```python
from build123d import *

# Parameters (mm, degrees)
F0_R     = 12.5
F0_R_2   = 2.55
F1_DEPTH = 6


# Not quite as in the source:
# - ends of sketch curves that miss each other by under 0.0002 mm in the source are joined


with BuildPart() as f1:
    # F0 (on Top) → F1 (new body)
    with BuildSketch(Plane.XY):
        with BuildLine():
            Line((38, 19.75), (-38, 19.75))
            ThreePointArc((-38, 19.75), (-40.1213203436, 18.8713203436), (-41, 16.75))
            Line((-41, 16.75), (-41, -16.75))
            ThreePointArc((-41, -16.75), (-40.1213203436, -18.8713203436), (-38, -19.75))
            Line((-38, -19.75), (38, -19.75))
            ThreePointArc((38, -19.75), (40.1213203436, -18.8713203436), (41, -16.75))
            Line((41, -16.75), (41, 16.75))
            ThreePointArc((41, 16.75), (40.1213203436, 18.8713203436), (38, 19.75))
        make_face()
        with BuildLine():
            ThreePointArc((-34.1539839892, -16.5960150108), (-36.3460155108, -16.5960155108), (-36.3460150108, -14.4039839892))
            Line((-36.346015, -14.403984), (-33.846015, -11.903984))
            ThreePointArc((-33.8460150108, -11.9039839892), (-31.6539844892, -11.9039844892), (-31.6539839892, -14.0960150108))
            Line((-31.653984, -14.096015), (-34.153984, -16.596015))
        make_face(mode=Mode.SUBTRACT)
        with BuildLine():
            ThreePointArc((-3.1539844892, -14.4039844892), (-3.1539844892, -16.5960155108), (-5.3460155108, -16.5960155108))
            Line((-5.3460155108, -16.5960155108), (-7.846015, -14.096015))
            ThreePointArc((-7.846015, -14.096015), (-7.8460155108, -11.9039844892), (-5.6539844892, -11.9039844892))
            Line((-5.6539844892, -11.9039844892), (-3.1539844892, -14.4039844892))
        make_face(mode=Mode.SUBTRACT)
        with Locations((-19.25, 0)):
            Circle(F0_R, mode=Mode.SUBTRACT)
        with Locations((12.8, -10)):
            Circle(F0_R_2, mode=Mode.SUBTRACT)
        with Locations((32.8, -10)):
            Circle(F0_R_2, mode=Mode.SUBTRACT)
        with Locations((12.8, 0)):
            Circle(F0_R_2, mode=Mode.SUBTRACT)
        with Locations((32.8, 0)):
            Circle(F0_R_2, mode=Mode.SUBTRACT)
        with BuildLine():
            ThreePointArc((-31.6539844892, 14.0960155108), (-31.6539844892, 11.9039844892), (-33.8460155108, 11.9039844892))
            Line((-33.8460155108, 11.9039844892), (-36.346015, 14.403985))
            ThreePointArc((-36.346015, 14.403985), (-36.3460155108, 16.5960155108), (-34.1539844892, 16.5960155108))
            Line((-34.1539844892, 16.5960155108), (-31.6539844892, 14.0960155108))
        make_face(mode=Mode.SUBTRACT)
        with BuildLine():
            ThreePointArc((-5.3460150108, 16.5960160108), (-3.1539844892, 16.5960155108), (-3.1539839892, 14.4039849892))
            Line((-3.153984, 14.403985), (-5.653984, 11.903985))
            ThreePointArc((-5.6539839892, 11.9039849892), (-7.8460155108, 11.9039844892), (-7.8460150108, 14.0960160108))
            Line((-7.846015, 14.096016), (-5.346015, 16.596016))
        make_face(mode=Mode.SUBTRACT)
        with Locations((12.8, 10)):
            Circle(F0_R_2, mode=Mode.SUBTRACT)
        with Locations((32.8, 10)):
            Circle(F0_R_2, mode=Mode.SUBTRACT)
    extrude(amount=F1_DEPTH)


solid = f1.part
```
Could you check a few things on this model? Use its own coordinates, in mm. A direction names the side the tool comes from. Round coordinates to 2 decimals unless told otherwise and drop trailing zeros. Loops run counter-clockwise (first coordinate to the right, second up) from the corner with the lowest first, then second, coordinate; pieces in that order, holes last. Notation, with made-up numbers: (-33.75, 45) -> (9.25, 45) arc R20 cw to (9.25, 79) -> close; hole circle Ø4 at (-37.5, 26.25). An arc over 180 degrees is marked (long way). One line per question, with ' | ' between items.
(1) For faces 1 (the face through (-4.42, -13.14, 2.96)), 2 (the face through (1, 19.75, 3)), which set-ups out of +Z, -Z, +X, -X, +Y, -Y let a thin tool reach every point of the face, with its end or its side?
Model answer:
face 1: +Z, -Z | face 2: +Z, -Z, +X, -X, +Y
(2) If we section it at D-D on x = -19.25: List the corners of the cut face in (y, z) for me, and give its area (3 significant figures).
Model answer:
outline: (-19.75, 0) -> (-12.5, 0) -> (-12.5, 6) -> (-19.75, 6) -> close; (12.5, 0) -> (19.75, 0) -> (19.75, 6) -> (12.5, 6) -> close | area: 87.0 mm^2
(3) Thinking about a two-plate mould opening in X: for faces 3 (the face through (-6.58, -15.36, 2.96)), 4 (the face through (-40.14, -18.85, 2.96)), 5 (the face through (-35.08, 13.14, 2.96)), 6 (the face through (41, 0, 3)), which applies, released by +X, released by -X, zero draft, split by the parting line, or undercut?
Model answer:
face 3: undercut | face 4: released by -X | face 5: undercut | face 6: released by +X
(4) If we section it at B-B on y = -10: List the corners of the cut face in (x, z) for me, and give its area (3 significant figures).
Model answer:
outline: (-41, 0) -> (-26.75, 0) -> (-26.75, 6) -> (-41, 6) -> close; (-11.75, 0) -> (10.25, 0) -> (10.25, 6) -> (-11.75, 6) -> close; (15.35, 0) -> (30.25, 0) -> (30.25, 6) -> (15.35, 6) -> close; (35.35, 0) -> (41, 0) -> (41, 6) -> (35.35, 6) -> close | area: 341 mm^2
(5) If we section it at A-A on x = 12.8: List the corners of the cut face in (y, z) for me, and give its area (3 significant figures).
Model answer:
outline: (-19.75, 0) -> (-12.55, 0) -> (-12.55, 6) -> (-19.75, 6) -> close; (-7.45, 0) -> (-2.55, 0) -> (-2.55, 6) -> (-7.45, 6) -> close; (2.55, 0) -> (7.45, 0) -> (7.45, 6) -> (2.55, 6) -> close; (12.55, 0) -> (19.75, 0) -> (19.75, 6) -> (12.55, 6) -> close | area: 145 mm^2
(6) If we section it at C-C on z = 3.1: Count the separate pieces of the cut face and the enclosed holes in it, and give its area (3 significant figures).
Model answer:
separate pieces: 1 | enclosed holes: 11 | area: 2,540 mm^2
(7) If I drill on probe 1 along Y at (x, z) = (12.8, 4.2); probe 2 along X at (y, z) = (14, 1.2); probe 3 along Y at (x, z) = (31, 1.9), over which ranges is the centre line in solid material (lowest first)?
Model answer:
probe 1: y = -19.75 to -12.55, -7.45 to -2.55, 2.55 to 7.45, 12.55 to 19.75 | probe 2: x = -41 to -35.94, -31.57 to -7.93, -3.56 to 41 | probe 3: y = -19.75 to -11.81, -8.19 to -1.81, 1.81 to 8.19, 11.81 to 19.75
